Geometry: see drawing. Coordinates: mm, zero at the bounding-box minimum. Coordinates: 2 decimals unless noted, no trailing zeros. Loops run counter-clockwise (first coordinate to the right, second up) from the corner with the lowest first, then second, coordinate; pieces in that order, holes last. Notation, with made-up numbers: (68, 8.25) -> (117, 8.25) arc R9 cw to (117, 19.25) -> close; hole circle Ø4 at (78.25, -3). An arc over 180 degrees is marked (long way). Answer as a JSON object with one key per item and string values.
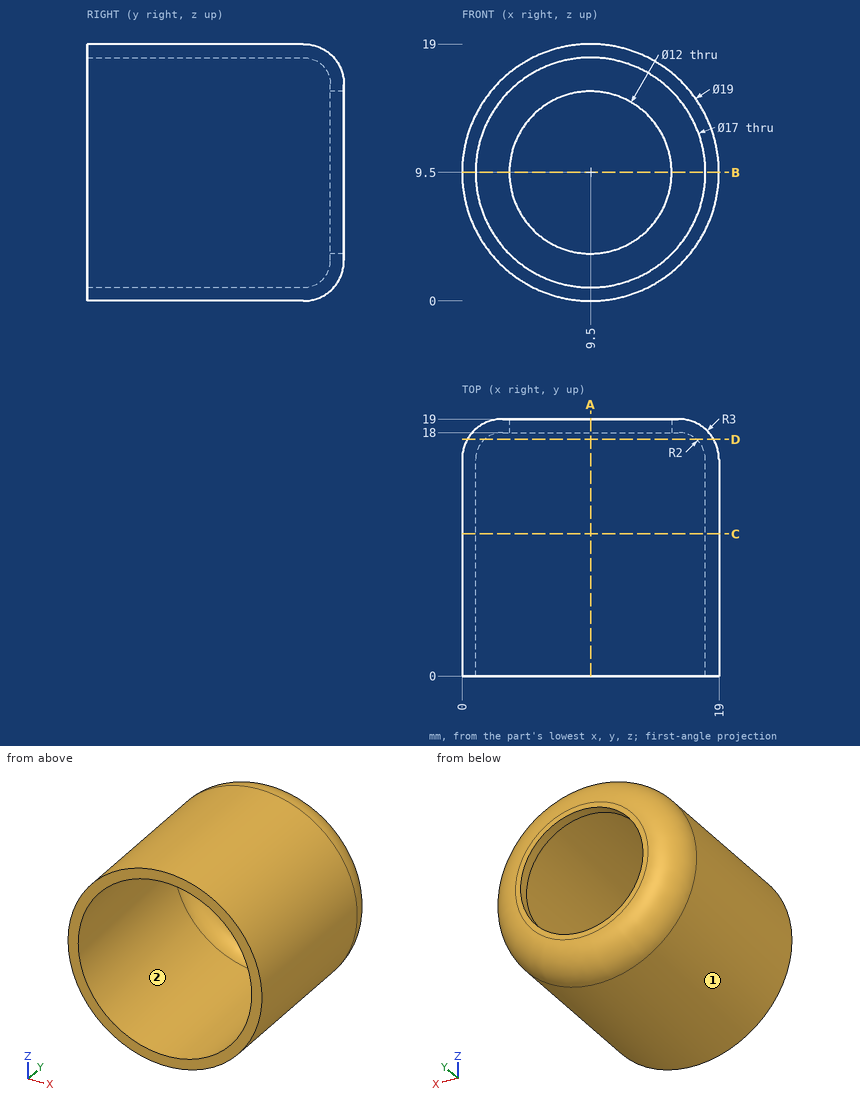
1. Line query: line 1 along Z through (x, y) = (9.5, 5.5); line 2 along X through (y, z) = (18.45, 9.5); line 3 along Z through (x, y) = (5.5, 10.5). Output: solid intervals per line, ascending.
Reply:
{"line 1": "z = 0 to 1, 18 to 19", "line 2": "x = 1.27 to 3.5, 15.5 to 17.73", "line 3": "z = 0.88 to 2, 17 to 18.12"}
2. Section query B-B (z = 9.5). Return loops of the section in (x, y).
Reply:
{"outline": "(0, 0) -> (1, 0) -> (1, 16) arc R2 cw to (3, 18) -> (3.5, 18) -> (3.5, 19) -> (3, 19) arc R3 ccw to (0, 16) -> close; (15.5, 18) -> (16, 18) arc R2 cw to (18, 16) -> (18, 0) -> (19, 0) -> (19, 16) arc R3 ccw to (16, 19) -> (15.5, 19) -> close"}
3. Mould query, pull axis X, two halves, no side actions, for the marked faces 1 and 2. Classes: pulls with the +X half, pulls with the -X half, needs draft (parallel to the pull), parting line crosses it, or undercut.
Reply:
{"face 1": "parting line crosses it", "face 2": "undercut"}
4. Section query A-A (x = 9.5). Return loops of the section in (y, z).
Reply:
{"outline": "(0, 0) -> (16, 0) arc R3 ccw to (19, 3) -> (19, 3.5) -> (18, 3.5) -> (18, 3) arc R2 cw to (16, 1) -> (0, 1) -> close; (0, 18) -> (16, 18) arc R2 cw to (18, 16) -> (18, 15.5) -> (19, 15.5) -> (19, 16) arc R3 ccw to (16, 19) -> (0, 19) -> close"}
5. Section query C-C (y = 10.5). Return loops of the section in (x, z).
Reply:
{"outline": "circle Ø19 at (9.5, 9.5); hole circle Ø17 at (9.5, 9.5)"}
6. Section query D-D (y = 17.5). Return loops of the section in (x, z), plus the area to 3 significant figures.
Reply:
{"outline": "circle Ø18.2 at (9.5, 9.5); hole circle Ø15.65 at (9.5, 9.5)", "area": "67.8 mm2"}
7. Pin query (flat end, axial travel): P1, Ø6, axis at x = 11, z = 2, coming from the -Y side; P2, Ø10, axis at x = 15, y = 8.5, coming from the +Z side; P3, Ø1.5, axis at x = 12, y = 7.5, coming from the +Z side; P4, Ø3, axis at y = 15.5, z = 15, coming from the -X side. Return the tip coordinate at first contact, or that it passes through.
Reply:
{"P1": "stops at y = 0", "P2": "stops at z = 18.99", "P3": "stops at z = 18.84", "P4": "stops at x = 0.88"}
